from build123d import *

# Parameters (mm, degrees)
SKETCH1_W           = 195
SKETCH1_H           = 67
BOSS_EXTRUDE1_DEPTH = 20
SKETCH2_R           = 6
CUT_EXTRUDE1_DEPTH  = 20
CUT_EXTRUDE2_DEPTH  = 120.980206701
CUT_EXTRUDE3_START  = -13
SKETCH4_W           = 3.612655346
SKETCH4_H           = 3
CUT_EXTRUDE3_DEPTH  = 13
SKETCH6_R           = 2.5
CUT_EXTRUDE4_DEPTH  = 106.016665344
SKETCH7_W           = 37
SKETCH7_H           = 35
CUT_EXTRUDE5_DEPTH  = 1.5


with BuildPart() as part:
    # Sketch1 → Boss-Extrude1 (new body)
    with BuildSketch(Plane(origin=(0, 0, 0), x_dir=(1, 0, 0), z_dir=(0, 1, 0))):
        Rectangle(SKETCH1_W, SKETCH1_H)
    extrude(amount=BOSS_EXTRUDE1_DEPTH)

    # Sketch2 → Cut-Extrude1 (cut)
    with BuildSketch(Plane.XZ):
        with BuildLine():
            Line((97.5, -3.219751644), (97.5, 33.5))
            Line((97.5, 33.5), (88.5, 33.5))
            ThreePointArc((88.5, 33.5), (95.217186872, 15.683556008), (97.5, -3.219751644))
        make_face()
        with BuildLine():
            Line((97.5, -33.5), (97.5, -3.219751644))
            ThreePointArc((97.5, -3.219751644), (95.985558513, -18.65423771), (91.5, -33.5))
            Line((91.5, -33.5), (97.5, -33.5))
        make_face()
        with BuildLine():
            ThreePointArc((-88, -33.5), (-95.08607052, -15.861694529), (-97.5, 2.992884749))
            Line((-97.5, 2.992884749), (-97.5, -33.5))
            Line((-97.5, -33.5), (-88, -33.5))
        make_face()
        with BuildLine():
            ThreePointArc((-97.5, 2.992884749), (-95.856964648, 18.588830376), (-91, 33.5))
            Line((-91, 33.5), (-97.5, 33.5))
            Line((-97.5, 33.5), (-97.5, 2.992884749))
        make_face()
        with Locations((31.9, -36.5)):
            Circle(SKETCH2_R)
    extrude(amount=-CUT_EXTRUDE1_DEPTH, mode=Mode.SUBTRACT)

    # Sketch3 → Cut-Extrude2 (cut, through all)
    with BuildSketch(Plane(origin=(0, 0, 33.5), x_dir=(-1, 0, 0), z_dir=(0, 0, -1))):
        Polygon((63.2, 20), (63.2, 9.6), (40.2, 9.6), (40.2, 5.6), (-61.8, 5.6), (-61.8, 9.6), (-97.5, 9.6), (-97.5, 20), align=None)
    extrude(amount=CUT_EXTRUDE2_DEPTH, mode=Mode.SUBTRACT)

    # Sketch4 → Cut-Extrude3 (cut)
    with BuildSketch(Plane(origin=(0, 20, 0), x_dir=(1, 0, 0), z_dir=(0, 1, 0)).offset(CUT_EXTRUDE3_START)):
        with BuildLine():
            Line((-63.2, 30.5), (-63.2, 33.5))
            Line((-63.2, 33.5), (-88, 33.5))
            ThreePointArc((-88, 33.5), (-88.810680862, 32.008999469), (-89.587344654, 30.5))
            Line((-89.587344654, 30.5), (-63.2, 30.5))
        make_face()
        with Locations((-61.393672327, 32)):
            Rectangle(SKETCH4_W, SKETCH4_H)
        with BuildLine():
            Line((-63.2, -33.5), (-63.2, -30.5))
            Line((-63.2, -30.5), (-92.261692194, -30.5))
            ThreePointArc((-92.261692194, -30.5), (-91.647155152, -32.006859002), (-91, -33.5))
            Line((-91, -33.5), (-63.2, -33.5))
        make_face()
        with Locations((-61.393672327, -32)):
            Rectangle(SKETCH4_W, SKETCH4_H)
    extrude(amount=CUT_EXTRUDE3_DEPTH, mode=Mode.SUBTRACT)

    # Sketch6 → Cut-Extrude4 (cut, through all)
    with BuildSketch(Plane.XZ):
        with Locations(Location((-28.1, -9, 0), (0, 0, 270))):
            Circle(SKETCH6_R)
        with Locations(Location((-8.2, -8.3, 0), (0, 0, 270))):
            Circle(SKETCH6_R)
        with Locations(Location((-18.7, 8.7, 0), (0, 0, 270))):
            Circle(SKETCH6_R)
        with Locations(Location((-76.2, 22, 0), (0, 0, 270))):
            Circle(SKETCH6_R)
        with Locations(Location((-78.2, 0.1, 0), (0, 0, 270))):
            Circle(SKETCH6_R)
        with Locations(Location((-73.2, -22.3, 0), (0, 0, 270))):
            Circle(SKETCH6_R)
        with Locations(Location((65.3, -20, 0), (0, 0, 270))):
            Circle(SKETCH6_R)
        with Locations(Location((74.1, -1.7, 0), (0, 0, 270))):
            Circle(SKETCH6_R)
        with Locations(Location((68.3, 21.5, 0), (0, 0, 270))):
            Circle(SKETCH6_R)
    extrude(amount=-CUT_EXTRUDE4_DEPTH, mode=Mode.SUBTRACT)

    # Sketch7 → Cut-Extrude5 (cut)
    with BuildSketch(Plane(origin=(0, 5.6, 0), x_dir=(1, 0, 0), z_dir=(0, 1, 0))):
        with Locations((5.3, -16)):
            Rectangle(SKETCH7_W, SKETCH7_H)
    extrude(amount=-CUT_EXTRUDE5_DEPTH, mode=Mode.SUBTRACT)


solid = part.part
Work out the finished part from the listing and answer in its coordinate system (mm). A direction names the side the tool comes from. Round coordinates to 2 decimals unless told otherwise and drop trailing zeros. Write each loop counter-clockwise with the first axis right and the second up, starting at its lowest first coordinate (ties: lowest second). Pieces come first, ordered by that corner, then holes.
1) A cutting plane is placed at C-C (x = 7). Give the vertices of the cut face in (y, z).
2) Given pin 1 Ø1.5 at (x, z) = (-68, -32.5) entering from +Y; pin 2 Ø0.8 at (x, y) = (4.5, 5) entering from +Z; pin 3 Ø6 at (x, z) = (-8.2, -8.3) entering from +Y; pin 4 Ø8 at (x, y) = (62, 15) entering from -Z, each flat-ended and moving along its own axis, determine where each tip first touches the part or whether it passes through.
3) A cutting plane is placed at D-D (z = 14). Give the vertices of the cut face in (x, y).
4) The mould has two halves that part along X. Classify faces 1 (the flat face through (-63.2, 15, 0)), 2 (the cylindrical face through (-25.62, 2.76, -8.67)), 3 (the flat face through (-2.5, 3.7, 33.5)): pulls with the +X half, pulls with the -X half, needs draft (parallel to the pull), parting line crosses it, or undercut.
5) Straight lines are drawn through the part: line 1 (X direction, y = 6, z = -22.3); line 2 (X direction, y = 9.5, z = 0.1); line 3 (X direction, y = 4, z = 21.5). For each, find the intervals that lie inside material, in ascending order.
6) A cutting plane is placed at A-A (z = 22). Give the vertices of the cut face in (x, y), plus the area to 3 significant figures.
7) A cutting plane is placed at B-B (y = 15). Give the vertices of the cut face in (x, z), plus the area to 3 significant figures.
8) A tool of negligible diameter and unlimited length cuts with its end or side. For faces 4 (the cylindrical face through (32, 2.8, -30.5)), 5 (the cylindrical face through (-75.72, 9.86, 0.43)), 6 (the flat face through (-76, 13, 30.5)), 7 (the flat face through (61.8, 8, 0)), 8 (the flat face through (79, 9.6, 0)), from which of +Z, -Z, +X, -X, +Y, -Y can it reach the whole face along a straight path? Write none if from no direction.
Completed:
1. outline: (0, -33.5) - (5.6, -33.5) - (5.6, -1.5) - (4.1, -1.5) - (4.1, 33.5) - (0, 33.5) - close
2. pin 1: stops at y = 7
2. pin 2: stops at z = -1.5
2. pin 3: stops at y = 5.6
2. pin 4: passes through
3. outline: (-96.69, 0) - (95.61, 0) - (95.61, 9.6) - (61.8, 9.6) - (61.8, 5.6) - (23.8, 5.6) - (23.8, 4.1) - (-13.2, 4.1) - (-13.2, 5.6) - (-40.2, 5.6) - (-40.2, 9.6) - (-63.2, 9.6) - (-63.2, 20) - (-96.69, 20) - close
4. face 1: pulls with the +X half
4. face 2: undercut
4. face 3: needs draft
5. line 1: x = -93.1 to -75.7, -70.7 to -40.2, 61.8 to 64.32, 66.28 to 95.17
5. line 2: x = -97.44 to -80.7, -75.7 to -40.2, 61.8 to 72.37, 75.83 to 97.43
5. line 3: x = -95.18 to -78.65, -73.75 to 65.8, 70.8 to 93.55
6. outline: (-95.05, 0) - (-78.7, 0) - (-78.7, 20) - (-95.05, 20) - close; (-73.7, 0) - (65.85, 0) - (65.85, 9.6) - (61.8, 9.6) - (61.8, 5.6) - (23.8, 5.6) - (23.8, 4.1) - (-13.2, 4.1) - (-13.2, 5.6) - (-40.2, 5.6) - (-40.2, 9.6) - (-63.2, 9.6) - (-63.2, 20) - (-73.7, 20) - close; (70.75, 0) - (93.39, 0) - (93.39, 9.6) - (70.75, 9.6) - close
6. area: 1,530 mm2
7. outline: (-92.26, 30.5) arc R74.84 ccw to (-89.59, -30.5) - (-63.2, -30.5) - (-63.2, 30.5) - close; hole circle Ø5 at (-78.2, 0.1); hole circle Ø5 at (-76.2, 22); hole circle Ø5 at (-73.2, -22.3)
7. area: 1,900 mm2
8. face 4: -Z, +Y, -Y
8. face 5: +Y, -Y
8. face 6: +Z, -X, +Y
8. face 7: +Z, -Z, +Y
8. face 8: +Z, -Z, +X, +Y
